Could you check a few things on this model? Use its own coordinates, in mm. A direction names the side the tool comes from. Round coordinates to 2 decimals unless told otherwise and drop trailing zeros. Loops run counter-clockwise (first coordinate to the right, second up) from the corner with the lowest first, then second, coordinate; pieces in that order, holes last. Notation, with made-up numbers: M 37.5,48 L 85.5,48 A25 ccw 85.5,68 Z; hole C 46,83 d11. An arc over 180 degrees is marked long. Answer in a Markdown table with one row per item.
```python
from build123d import *

# Parameters (mm, degrees)
SKETCH1_R           = 2.07
SKETCH1_R_2         = 6.07
BOSS_EXTRUDE1_DEPTH = 1.5
FILLET1_R           = 3


with BuildPart() as part:
    # Sketch1 → Boss-Extrude1 (new, symmetric)
    # profile 1 of 5: a face of its own
    with BuildSketch(Plane.XY):
        with BuildLine():
            ThreePointArc((6.07, 25.4), (0, 19.33), (-6.07, 25.4))
            Line((-6.07, 25.4), (-6.07, 0))
            ThreePointArc((-6.07, 0), (0, 6.07), (6.07, 0))
            Line((6.07, 0), (6.07, 6.07))
            Line((6.07, 6.07), (6.07, 25.4))
        make_face()
        with Locations((0, 12.7)):
            Circle(SKETCH1_R, mode=Mode.SUBTRACT)
    # profile 2 of 5: a face of its own
    with BuildSketch(Plane.XY):
        with Locations((0, 25.4)):
            Circle(SKETCH1_R_2)
        with Locations((0, 25.4)):
            Circle(SKETCH1_R, mode=Mode.SUBTRACT)
    # profile 3 of 5: a face of its own
    with BuildSketch(Plane.XY):
        Circle(SKETCH1_R_2)
        Circle(SKETCH1_R, mode=Mode.SUBTRACT)
    # profile 4 of 5: a face of its own
    with BuildSketch(Plane.XY):
        with BuildLine():
            Line((6.07, 6.07), (6.07, 0))
            ThreePointArc((6.07, 0), (4.292138162, -4.292138162), (0, -6.07))
            Line((0, -6.07), (25.4, -6.07))
            ThreePointArc((25.4, -6.07), (19.33, 0), (25.4, 6.07))
            Line((25.4, 6.07), (6.07, 6.07))
        make_face()
        with Locations((12.7, 0)):
            Circle(SKETCH1_R, mode=Mode.SUBTRACT)
    # profile 5 of 5: a face of its own
    with BuildSketch(Plane.XY):
        with Locations((25.4, 0)):
            Circle(SKETCH1_R_2)
        with Locations((25.4, 0)):
            Circle(SKETCH1_R, mode=Mode.SUBTRACT)
    extrude(amount=BOSS_EXTRUDE1_DEPTH, both=True)

    # Fillet1
    fillet1_edges = [part.edges().sort_by_distance(p)[0] for p in [
        (6.07, 6.07, 0),
    ]]
    fillet(fillet1_edges, radius=FILLET1_R)


solid = part.part
```
1) If we mould it in two halves opening along Z, with no side actions, what happens to faces 1 (the face through (4, 9, 1.5)), 2 (the face through (4, 9, -1.5)), 3 (the face through (31.47, -0.13, 0.02))? For each: released by +Z, released by -Z, zero draft, split by the parting line, or undercut.
Computed:
| item | result |
|---|---|
| face 1 | released by +Z |
| face 2 | released by -Z |
| face 3 | zero draft |
2) I want a section at C-C, the plane y = 14. Please give me the cut outline in (x, z), plus the area to 3 significant figures.
Computed:
| item | result |
|---|---|
| outline | M -6.07,-1.5 L -1.61,-1.5 L -1.61,1.5 L -6.07,1.5 Z; M 1.61,-1.5 L 6.07,-1.5 L 6.07,1.5 L 1.61,1.5 Z |
| area | 26.8 mm² |
3) Will these pins go through, and if not, where does the flat tip stop? P1, Ø3.5, axis at x = 12.7, y = 0, coming from the +Z side; P2, Ø0.9, axis at x = 21, z = 0.5, coming from the +Y side.
Computed:
| item | result |
|---|---|
| P1 | passes through |
| P2 | stops at y = 6.07 |
4) I want a section at A-A, the plane x = 12.7. Please give me the cut outline in (y, z).
Computed:
| item | result |
|---|---|
| outline | M -6.07,-1.5 L -2.07,-1.5 L -2.07,1.5 L -6.07,1.5 Z; M 2.07,-1.5 L 6.07,-1.5 L 6.07,1.5 L 2.07,1.5 Z |
5) Which directions (+Z, -Z, +X, -X, +Y, -Y) give clear straight access to the entire face, cutting with the end or side of a thin tool? Please do faces 4 (the face through (13, -6.07, 0)), 5 (the face through (17, 6.07, 0)).
Computed:
| item | result |
|---|---|
| face 4 | +Z, -Z, +X, -X, -Y |
| face 5 | +Z, -Z, +X, +Y |
6) I need wall thicknesses on line 1 (X direction, y = 20, z = 1.3); line 2 (Y direction, x = 12.7, z = 0.6); line 3 (X direction, y = 26.5, z = 1.2). Which ranges of each line are inside material? Lowest first, please.
Computed:
| item | result |
|---|---|
| line 1 | x = -6.07 to 6.07 |
| line 2 | y = -6.07 to -2.07, 2.07 to 6.07 |
| line 3 | x = -5.97 to -1.75, 1.75 to 5.97 |
7) I want a section at B-B, the plane z = -1. Please give me the cut outline in (x, y), plus the area to 3 significant figures.
Computed:
| item | result |
|---|---|
| outline | M -6.07,0 A6.07 ccw 0,-6.07 L 25.4,-6.07 A6.07 ccw 25.4,6.07 L 9.07,6.07 A3 cw 6.07,9.07 L 6.07,25.4 A6.07 ccw -6.07,25.4 Z; hole C 0,0 d4.14; hole C 0,12.7 d4.14; hole C 0,25.4 d4.14; hole C 12.7,0 d4.14; hole C 25.4,0 d4.14 |
| area | 659 mm² |
8) I want a section at D-D, the plane y = 3. Please give me the cut outline in (x, z).
Computed:
| item | result |
|---|---|
| outline | M -6.07,-1.5 L 30.68,-1.5 L 30.68,1.5 L -6.07,1.5 Z |
